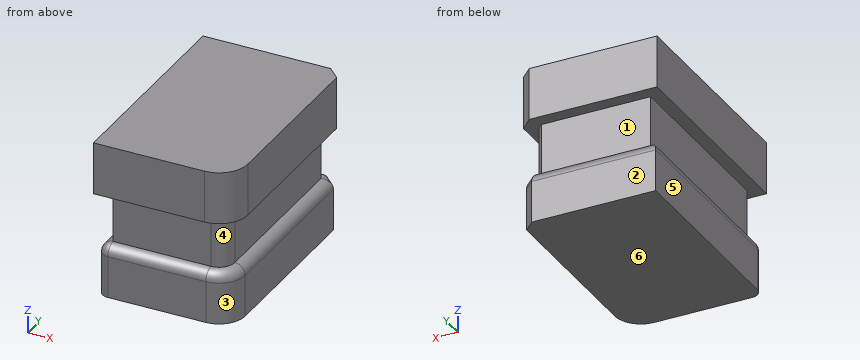
```python
from build123d import *

# Parameters (mm, degrees)
F0_W     = 65.419092
F0_H     = 101.706258
F1_DEPTH = 25.4
F2_SIZE  = 5.08
F3_R     = 5.08
F4_R     = 12.7
F5_R     = 5.08
F6_DEPTH = 25.4
F8_DEPTH = 25.4


with BuildPart() as f1:
    # F0 (on Top) → F1 (new body)
    with BuildSketch(Plane.XY):
        Rectangle(F0_W, F0_H)
    extrude(amount=F1_DEPTH)

    # F2
    f2_edges = [f1.edges().sort_by_distance(p)[0] for p in [
        (32.709546, 50.853129, 12.7),
    ]]
    chamfer(f2_edges, length=F2_SIZE)

    # F3
    f3_edges = [f1.edges().sort_by_distance(p)[0] for p in [
        (-32.709546, -50.853129, 12.7),
    ]]
    fillet(f3_edges, radius=F3_R)

    # F4
    f4_edges = [f1.edges().sort_by_distance(p)[0] for p in [
        (32.709546, -50.853129, 12.7),
    ]]
    fillet(f4_edges, radius=F4_R)

    # F5
    f5_edges = [f1.edges().sort_by_distance(p)[0] for p in [
        (32.709546, 3.81, 25.4),
        (-3.81, -50.853129, 25.4),
        (28.989803, -47.133386, 25.4),
        (-31.221649, -49.365232, 25.4),
        (-32.709546, 2.54, 25.4),
        (30.169546, 48.313129, 25.4),
        (-2.54, 50.853129, 25.4),
    ]]
    fillet(f5_edges, radius=F5_R)

    # F1_face (on face) → F6 (join)
    with BuildSketch(Plane(origin=(-0.075869, 0.08909, 25.4), x_dir=(1, 0, 0), z_dir=(0, 0, 1))):
        with BuildLine():
            Line((-27.553677, 45.68404), (-27.553677, -45.862219))
            Line((-27.553677, -45.862219), (20.085415, -45.862219))
            ThreePointArc((20.085415, -45.862219), (25.473569, -43.630373), (27.705415, -38.242219))
            Line((27.705415, -38.242219), (27.705415, 43.579835))
            Line((27.705415, 43.579835), (25.60121, 45.68404))
            Line((25.60121, 45.68404), (-27.553677, 45.68404))
        make_face()
    extrude(amount=F6_DEPTH)

    # F7 (on face) → F8 (join)
    with BuildSketch(Plane.XY.offset(50.8)):
        with BuildLine():
            Line((28.155598, 52.123129), (-33.979546, 52.123129))
            Line((-33.979546, 52.123129), (-33.979546, -52.123129))
            Line((-33.979546, -52.123129), (20.009546, -52.123129))
            ThreePointArc((20.009546, -52.123129), (29.887828, -48.031411), (33.979546, -38.153129))
            Line((33.979546, -38.153129), (33.979546, 46.299181))
            Line((33.979546, 46.299181), (28.155598, 52.123129))
        make_face()
    extrude(amount=F8_DEPTH)


solid = f1.part
```
CAD build for the part. Positions are in the model's coordinates, mm. Face numbers are marked on the shaded views. A direction names the side the tool comes from. Round coordinates to 2 decimals unless told otherwise and drop trailing zeros. Loops run counter-clockwise (first coordinate to the right, second up) from the corner with the lowest first, then second, coordinate; pieces in that order, holes last. Notation, with made-up numbers: (51.5, 69.5) - (68.5, 69.5) arc R17 ccw to (68.5, 82.5) - close; hole circle Ø5 at (-11.75, 28.25). An arc over 180 degrees is marked (long way). Return JSON: item names as keys, results as strings. Group by question number.
Q1. Band-saw the part on A-A on z = 46.5. Give the cut face in (x, y).
Q2. Two-plate mould, pull along Z, no slides. Class the marked faces 4, 5 and 6: +Z half, -Z half, draft (parallel to the pull), parting line (faces both ways), or undercut.
Q3. Band-saw the part on B-B on x = -6.5. Give the cut face in (y, z).
Q4. Band-saw the part on D-D on z = 11.5. Give the cut face in (x, y).
Q5. Flat gauge pins, fed straight in: pin 1 Ø7.5 at (y, z) = (6.5, 44.5) entering from +X; pin 2 Ø8 at (x, z) = (7.5, 12) entering from -Y; pin 3 Ø10 at (x, z) = (-4.5, 5.5) entering from +Y. Where does each tip first touch, or does it go through?
Q6. Band-saw the part on C-C on y = 23. Give the cut face in (x, z).
Q7. Tool access for the marked faces 1, 2 and 3: list every direction of +Z, -Z, +X, -X, +Y, -Y with a clear straight run to the whole face (end or side of a thin tool).
Q8. Drill centre lines: line 1 along Y through (x, z) = (18.5, 4.5); line 2 along Z through (x, y) = (-30, 44); line 3 along X through (y, z) = (-37, 30). Where is each one in solid material? Low to high. Write a range as [from, to].
Solutions:
{
 "1": {"outline": "(-27.63, -45.77) - (20.01, -45.77) arc R7.62 ccw to (27.63, -38.15) - (27.63, 43.67) - (25.53, 45.77) - (-27.63, 45.77) - close"},
 "2": {"face 4": "undercut", "face 5": "draft", "face 6": "-Z half"},
 "3": {"outline": "(-52.12, 50.8) - (-45.77, 50.8) - (-45.77, 25.4) arc R5.08 ccw to (-50.85, 20.32) - (-50.85, 0) - (50.85, 0) - (50.85, 20.32) arc R5.08 ccw to (45.77, 25.4) - (45.77, 50.8) - (52.12, 50.8) - (52.12, 76.2) - (-52.12, 76.2) - close"},
 "4": {"outline": "(-32.71, -45.77) arc R5.08 ccw to (-27.63, -50.85) - (20.01, -50.85) arc R12.7 ccw to (32.71, -38.15) - (32.71, 45.77) - (27.63, 50.85) - (-32.71, 50.85) - close"},
 "5": {"pin 1": "stops at x = 27.63", "pin 2": "stops at y = -50.85", "pin 3": "stops at y = 50.85"},
 "6": {"outline": "(-33.98, 50.8) - (-27.63, 50.8) - (-27.63, 25.4) arc R5.08 ccw to (-32.71, 20.32) - (-32.71, 0) - (32.71, 0) - (32.71, 20.32) arc R5.08 ccw to (27.63, 25.4) - (27.63, 50.8) - (33.98, 50.8) - (33.98, 76.2) - (-33.98, 76.2) - close"},
 "7": {"face 1": "+X, -X, +Y", "face 2": "-Z, +X, -X, +Y", "face 3": "-Z, +X, -Y"},
 "8": {"line 1": "y = [-50.85, 50.85]", "line 2": "z = [0, 24.81], [50.8, 76.2]", "line 3": "x = [-27.63, 27.63]"}
}
